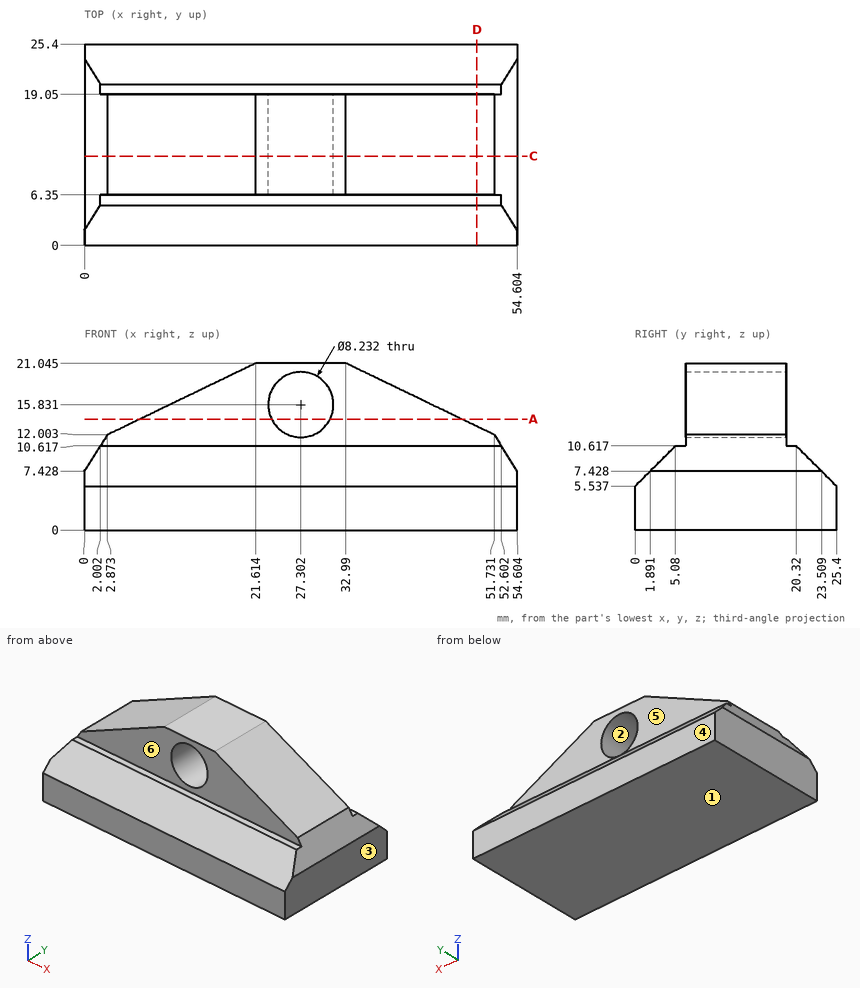
Geometry: see drawing. Coordinates: mm, zero at the bounding-box minimum. A direction names the side the tool comes from. Round coordinates to 2 decimals unless told otherwise and drop trailing zeros. Write each loop counter-clockwise with the first axis right and the second up, starting at its lowest first coordinate (ties: lowest second). Pieces come first, ordered by that corner, then holes. Notation, with made-up numbers: M 20.5,35.5 L 58.5,35.5 A35 cw 58.5,74.5 Z; hole C 60.25,79.25 d3. An arc over 180 degrees is marked long. Answer as a JSON object with one key per item and string values. Group by question number.
(1) Reachability of the marked faces 4, 5 and 6 from +Z, -Z, +X, -X, +Y, -Y: full face, straight path, thin tool, end or side. Return the list, or none.
(2) First-contact query: pin 1 (1 mm diameter, centred on y = 19.5, z = 6.5, fed in from -X); pin 2 (1.5 mm diameter, centred on x = 45, z = 11.5, fed in from -Y); pin 3 (6 mm diameter, centred on y = 3, z = 11, fed in from +X) (1 decimal); pin 4 (10.5 mm diameter, centred on x = 27.3, z = 15.83, fed in from +Y). Flat tips, straight axial feed; report the tip coordinate or a pass-through.
(3) Mould query, pull axis X, two halves, no side actions, for the marked faces 1, 2 and 3. Classes: +X half, -X half, draft (parallel to the pull), parting line (faces both ways), or undercut.
(4) Section query C-C on y = 11.25. Output: boundary loops of the cut face in (x, z) (1 decimal).
(5) Ray query, line 1 (Z direction, x = 49, y = 23.5) (1 decimal); line 2 (Z direction, x = 17.5, y = 14); line 3 (Y direction, x = 38, z = 18.5). Return the intervals inside material, ascending. Write a range as [from, to].
(6) Section query D-D on x = 49.5. Output: boundary loops of the cut face in (y, z), then the cut area to 3 significant figures.
(7) Section query A-A on z = 14. Output: boundary loops of the cut face in (x, y), then the cut area to 3 significant figures.
Computed values:
{
 "1": {"face 4": "+Z, -Z, +X, -X, +Y", "face 5": "+Z, +X, -X, +Y", "face 6": "+Z, +X, -X, -Y"},
 "2": {"pin 1": "x = 0", "pin 2": "y = 6.35", "pin 3": "x = 54.2", "pin 4": "y = 20.36"},
 "3": {"face 1": "draft", "face 2": "undercut", "face 3": "+X half"},
 "4": {"outline": "M 0,0 L 54.6,0 L 54.6,7.4 L 51.7,12 L 33,21 L 21.6,21 L 2.9,12 L 0,7.4 Z; hole C 27.3,15.8 d8.2"},
 "5": {"line 1": "[0, 7.4]", "line 2": "[0, 19.06]", "line 3": "[6.35, 19.05]"},
 "6": {"outline": "M 0,0 L 25.4,0 L 25.4,5.54 L 20.32,10.62 L 19.05,10.62 L 19.05,13.08 L 6.35,13.08 L 6.35,10.62 L 5.08,10.62 L 0,5.54 Z", "area": "275 mm^2"},
 "7": {"outline": "M 7.01,6.35 L 23.62,6.35 L 23.62,19.05 L 7.01,19.05 Z; M 30.99,6.35 L 47.59,6.35 L 47.59,19.05 L 30.99,19.05 Z", "area": "422 mm^2"}
}
